The listing builds one solid part. Answer for the finished solid, in the listing's coordinates (mm). A direction names the side the tool comes from. Round coordinates to 2 decimals unless told otherwise and drop trailing zeros. Loops run counter-clockwise (first coordinate to the right, second up) from the corner with the lowest first, then second, coordinate; pieces in that order, holes last. Notation, with made-up numbers: (30.5, 85) -> (62.5, 85) arc R31 cw to (62.5, 124) -> close; hole circle Ø9 at (60.5, 47). An arc over 180 degrees is marked (long way). Write each question's results on one line, items separated by ' | '. Start each with the question number.
(1) The part is cut by section C-C (y = -9). Determine the outline of the cut face in (x, z).
(2) Determine the mould class of faces 1 (the face through (-25.4, 0, 0)), 2 (the face through (-6, -12, -25.4)), 3 (the face through (-10.1, -15.3, -7.7)), 4 (the face through (-9.36, 15.7, 8.583)) for opening direction Z: released by +Z, released by -Z, zero draft, split by the parting line, or undercut.
(3) Flat-ended cylindrical pins translate along their axes: pin 1 (1.5 mm diameter, centred on x = 35.5, z = 3.5, fed in from -Y); pin 2 (4 mm diameter, centred on y = 15.5, z = -14.5, fed in from +X); pin 3 (12 mm diameter, centred on x = 1, y = -8.5, fed in from +Z). Find the tip coordinate at first contact, or state that the pin passes through.
(4) The part is cut by section B-B (z = 18). Determine the outline of the cut face in (x, y), plus the area to 3 significant figures.
(5) Straight lines are drawn through the part: probe 1 along X at (y, z) = (15, 0); probe 2 along X at (y, z) = (0, 9). For each, find the intervals that lie inside material, in ascending order.
(6) The part is cut by section A-A (x = 0). Determine the outline of the cut face in (y, z), plus the area to 3 significant figures.
(7) For faces 5 (the face through (25.4, -12, -6)), 6 (the face through (-6, -25.4, 12)), determine the directions among +Z, -Z, +X, -X, +Y, -Y from which every point of the face is accessible in a straight line to the end or side of a thin tool.
```python
from build123d import *

# Parameters (mm, degrees)
F0_W     = 50.8
F0_H     = 50.8
F0_R     = 12.7
F1_DEPTH = 25.4
F2_R     = 12.7
F3_DEPTH = 50.801
F4_R     = 12.7
F5_DEPTH = 25.4


with BuildPart() as f1:
    # F0 (on Front) → F1 (new body, symmetric)
    with BuildSketch(Plane.XZ):
        Rectangle(F0_W, F0_H)
        Circle(F0_R, mode=Mode.SUBTRACT)
    extrude(amount=F1_DEPTH, both=True)

    # F2 (on face) → F3 (cut, through all)
    with BuildSketch(Plane.XY.offset(25.4)):
        Circle(F2_R)
    extrude(amount=-F3_DEPTH, mode=Mode.SUBTRACT)

    # F4 (on face) → F5 (join)
    with BuildSketch(Plane.YZ.offset(25.4)):
        Circle(F4_R)
    extrude(amount=F5_DEPTH)


solid = f1.part
```
Checked values:
1) outline: (-25.4, -25.4) -> (-8.96, -25.4) -> (-8.96, -9) arc R12.7 cw to (-8.96, 9) -> (-8.96, 25.4) -> (-25.4, 25.4) -> close; (8.96, -25.4) -> (25.4, -25.4) -> (25.4, -8.96) -> (50.8, -8.96) -> (50.8, 8.96) -> (25.4, 8.96) -> (25.4, 25.4) -> (8.96, 25.4) -> (8.96, 9) arc R12.7 cw to (8.96, -9) -> close
2) face 1: zero draft | face 2: released by -Z | face 3: undercut | face 4: undercut
3) pin 1: stops at y = -12.4 | pin 2: stops at x = 25.4 | pin 3: stops at z = 25.4
4) outline: (-25.4, -25.4) -> (25.4, -25.4) -> (25.4, 25.4) -> (-25.4, 25.4) -> close; hole circle Ø25.4 at (0, 0) | area: 2,070 mm2
5) probe 1: x = -25.4 to -12.7, 12.7 to 25.4 | probe 2: x = -25.4 to -12.7, 12.7 to 50.8
6) outline: (-25.4, -25.4) -> (-12.7, -25.4) -> (-12.7, -12.7) -> (-25.4, -12.7) -> close; (-25.4, 12.7) -> (-12.7, 12.7) -> (-12.7, 25.4) -> (-25.4, 25.4) -> close; (12.7, -25.4) -> (25.4, -25.4) -> (25.4, -12.7) -> (12.7, -12.7) -> close; (12.7, 12.7) -> (25.4, 12.7) -> (25.4, 25.4) -> (12.7, 25.4) -> close | area: 645 mm2
7) face 5: +X | face 6: +Z, -Z, +X, -X, -Y
